```python
from build123d import *

# Parameters (mm, degrees)
SKETCH1_W           = 46
SKETCH1_H           = 6
BOSS_EXTRUDE1_DEPTH = 27.35
BOSS_EXTRUDE2_DEPTH = 27.35
FILLET1_R           = 7
BOSS_EXTRUDE3_DEPTH = 86
FILLET2_R           = 3
SKETCH5_R           = 8
SKETCH5_R_2         = 4
CUT_EXTRUDE1_DEPTH  = 116.185263628
SKETCH6_R           = 4
CUT_EXTRUDE2_DEPTH  = 116.185263741
SKETCH7_R           = 4
CUT_EXTRUDE3_DEPTH  = 116.185263741
SKETCH8_R           = 8
SKETCH8_R_2         = 4
BOSS_EXTRUDE4_DEPTH = 6
SKETCH9_R           = 8
SKETCH9_R_2         = 4
BOSS_EXTRUDE5_DEPTH = 6
SKETCH11_R          = 4
BOSS_EXTRUDE6_DEPTH = 3


with BuildPart() as part:
    # Sketch1 → Boss-Extrude1 (new body)
    with BuildSketch(Plane(origin=(0, 0, 0), x_dir=(0, 0, -1), z_dir=(1, 0, 0))):
        with Locations((1.147704591, 3)):
            Rectangle(SKETCH1_W, SKETCH1_H)
    extrude(amount=-BOSS_EXTRUDE1_DEPTH)

    # Sketch2 → Boss-Extrude2 (add)
    with BuildSketch(Plane(origin=(0, 0, 0), x_dir=(0, 0, -1), z_dir=(1, 0, 0))):
        Polygon((-21.852295409, 6), (-65.755273625, -10.778811155), (-63.703152765, -16.41696688), (-18.597906967, 0), align=None)
    extrude(amount=-BOSS_EXTRUDE2_DEPTH)

    # Fillet1
    fillet1_edges = [part.edges().sort_by_distance(p)[0] for p in [
        (-13.675, 6, 21.852295409),
    ]]
    fillet(fillet1_edges, radius=FILLET1_R)

    # Sketch3 → Boss-Extrude3 (add)
    with BuildSketch(Plane(origin=(0, 0, -24.147704591), x_dir=(-1, 0, 0), z_dir=(0, 0, -1))):
        with BuildLine():
            ThreePointArc((27.35, 6), (13.675, 19.675), (0, 6))
            Line((0, 6), (27.35, 6))
        make_face()
        with BuildLine():
            Line((25.963434603, 0), (1.386565397, 0))
            ThreePointArc((1.386565397, 0), (13.675, -7.675), (25.963434603, 0))
        make_face()
        with BuildLine():
            Line((27.35, 6), (0, 6))
            ThreePointArc((0, 6), (0.351149802, 2.920935061), (1.386565397, 0))
            Line((1.386565397, 0), (25.963434603, 0))
            ThreePointArc((25.963434603, 0), (26.998850198, 2.920935061), (27.35, 6))
        make_face()
    extrude(amount=BOSS_EXTRUDE3_DEPTH)

    # Fillet2
    # the kernel refuses this fillet: 3 mm, written as the material it adds along each edge
    with BuildSketch(Plane(origin=(0, 6, -24.147704591), x_dir=(0, 0, 1), z_dir=(-1, 0, 0))) as fillet2_piece_1_section:
        with BuildLine():
            CenterArc((FILLET2_R, FILLET2_R), FILLET2_R, 180, 90)
            Line((0, FILLET2_R), (0, 0))
            Line((0, 0), (FILLET2_R, 0))
        make_face()
    fillet2_piece_1 = extrude(amount=27.35, mode=Mode.PRIVATE)
    fillet2_piece_1 = fillet2_piece_1 & Plane(origin=(-13.675, 6, -23.467343504), x_dir=(-1, 0, 0), z_dir=(0, 0, 1)) * Cylinder(13.675, 67, mode=Mode.PRIVATE)
    add(fillet2_piece_1)

    # Sketch5 → Cut-Extrude1 (cut, through all)
    with BuildSketch(Plane(origin=(0, 0, 0), x_dir=(1, 0, 0), z_dir=(0, 1, 0))):
        with Locations(Location((-12.203148076, 67.147704591, 0), (0, 0, 259.398243128))):
            Circle(SKETCH5_R)
        with Locations(Location((-12.203148076, 67.147704591, 0), (0, 0, 248.409956221))):
            Circle(SKETCH5_R_2, mode=Mode.SUBTRACT)
    extrude(amount=CUT_EXTRUDE1_DEPTH, mode=Mode.SUBTRACT)

    # Sketch6 → Cut-Extrude2 (cut, through all)
    with BuildSketch(Plane(origin=(0, 0, 0), x_dir=(1, 0, 0), z_dir=(0, 1, 0))):
        with Locations((-12.203148076, 67.147704591)):
            Circle(SKETCH6_R)
    extrude(amount=CUT_EXTRUDE2_DEPTH, mode=Mode.SUBTRACT)

    # Sketch7 → Cut-Extrude3 (cut, through all)
    with BuildSketch(Plane(origin=(0, 0, 0), x_dir=(1, 0, 0), z_dir=(0, 1, 0))):
        with Locations(Location((-12.203148076, 67.147704591, 0), (0, 0, 270))):
            Circle(SKETCH7_R)
    extrude(amount=-CUT_EXTRUDE3_DEPTH, mode=Mode.SUBTRACT)

    # Sketch8 → Boss-Extrude4 (add)
    with BuildSketch(Plane(origin=(0, 0, 0), x_dir=(1, 0, 0), z_dir=(0, 1, 0))):
        with Locations(Location((-12.203148076, 67.147704591, 0), (0, 0, 259.398243128))):
            Circle(SKETCH8_R)
        with Locations(Location((-12.203148076, 67.147704591, 0), (0, 0, 270))):
            Circle(SKETCH8_R_2, mode=Mode.SUBTRACT)
    extrude(amount=BOSS_EXTRUDE4_DEPTH)

    # Sketch9 → Boss-Extrude5 (add)
    with BuildSketch(Plane(origin=(0, 6, 0), x_dir=(1, 0, 0), z_dir=(0, 1, 0))):
        with Locations(Location((-12.203148076, 67.147704591, 0), (0, 0, 259.398243128))):
            Circle(SKETCH9_R)
        with Locations(Location((-12.203148076, 67.147704591, 0), (0, 0, 270))):
            Circle(SKETCH9_R_2, mode=Mode.SUBTRACT)
    extrude(amount=BOSS_EXTRUDE5_DEPTH)


with BuildPart() as part_1:
    # Body-Move/Copy1: moved
    add(part.part.moved(Location((13.675, 0, 0))))

    # Sketch11 → Boss-Extrude6 (add, symmetric)
    with BuildSketch(Plane(origin=(0, 0, 0), x_dir=(0, 0, -1), z_dir=(1, 0, 0))):
        with BuildLine():
            Line((-65.755273625, -10.778811155), (-21.830832444, 5.883719563))
            Line((-21.830832444, 5.883719563), (-26.796391829, 18.97353316))
            ThreePointArc((-26.796391829, 18.97353316), (-28.894991358, 21.202538099), (-31.955069824, 21.294748649))
            Line((-31.955069824, 21.294748649), (-68.432005738, 7.457394118))
            ThreePointArc((-68.432005738, 7.457394118), (-70.663039196, 5.354278937), (-70.749698163, 2.289463448))
            Line((-70.749698163, 2.289463448), (-65.755273625, -10.778811155))
        make_face()
        with Locations((-43.013345846, 5.334970097)):
            Circle(SKETCH11_R, mode=Mode.SUBTRACT)
    extrude(amount=BOSS_EXTRUDE6_DEPTH, both=True)


solid = part_1.part
```
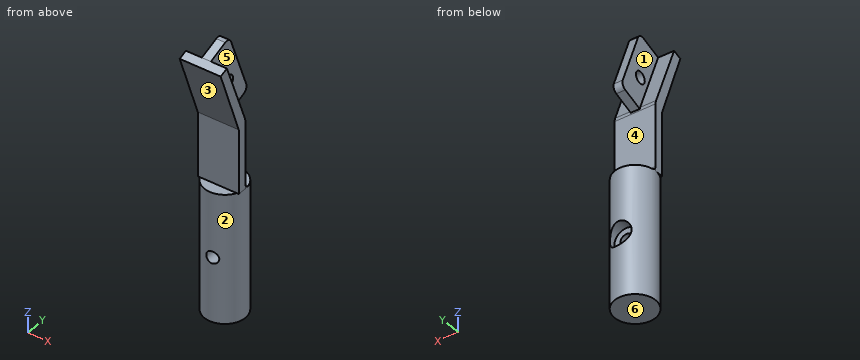
Input: part model. Units: mm. Frame: model coordinates. Face numbers are marked on the shaded views. A direction names the side the tool comes from. Give positions to 0.01 mm unless a question says otherwise; leave off trailing zeros. Write each loop counter-clockwise with the first axis right and the second up, starting at its lowest first coordinate (ties: lowest second). Pieces come first, ordered by that corner, then holes. Notation, with made-up numbers: (-13, 37) - (40, 37) arc R22 ccw to (40, 47) - close; hole circle Ø4 at (-37.75, 60.5). An arc over 180 degrees is marked (long way). Write item = value, one per line. Start each with the question number.
1) Reachability of the marked faces 1, 2 and 3 from +Z, -Z, +X, -X, +Y, -Y: full face, straight path, thin tool, end or side. Return the list, or none.
2) Cut plane D-D (x = -8.25). Return loops of the section in (y, z), and give its area (3 significant figures).
3) Cut plane B-B (y = 17). Return loops of the section in (x, z), and give its area (3 significant figures).
4) Cut plane C-C (z = -52). Return loops of the section in (x, y) (3 decimals), and give its area (3 significant figures).
5) Pin query (flat end, axial travel): pin 1 (2 mm diameter, centred on x = 7, y = -6.5, fed in from -Z); pin 2 (5 mm diameter, centred on x = 4, z = -21, fed in from -Y); pin 3 (10.5 mm diameter, centred on x = 1.47, z = -67.15, fed in from +Y); pin 4 (5 mm diameter, centred on x = 3.5, z = 34.5, fed in from -Y). Return the tip coordinate at first contact, or that it passes through.
6) Draft query along Z for the marked faces 4, 5 and 6. Return one class per face: pulls with the +Z half, pulls with the -Z half, needs draft (parallel to the pull), parting line crosses it, or undercut.
7) Material intervals for L1, parallel to X at y = 3, z = 34; L2, parallel to Z at x = -12, y = 11; L3, parallel to Y at x = 1, z = 18.5, sorted ascending. Write a range as [from, to].
8) Cut plane A-A (y = -4.5). Return loops of the section in (x, z) (3 decimals), and give its area (3 significant figures).
Answers follow:
q1.face_1 = +Z, -X, +Y
q1.face_2 = -Z
q1.face_3 = +X, -X, -Y
q2.outline = (-16.42, 63.7) - (0, 18.6) - (0, -24.15) - (-4.91, -24.15) - (-4.91, -110.15) - (16.91, -110.15) - (16.91, -24.15) - (9, -24.15) arc R3 cw to (6, -21.15) - (6, 20.56) arc R7 ccw to (5.54, 23.06) - (-10.78, 65.76) - close
q2.area = 2,450 mm^2
q3.outline = (-8.12, -110.15) - (8.12, -110.15) - (8.12, -71.59) arc R8 cw (long way) to (8.12, -62.7) - (8.12, -24.15) - (-8.12, -24.15) - close; (-3, 26.05) - (3, 26.05) - (3, 43.28) - (-3, 43.28) - close
q3.area = 1,310 mm^2
q4.outline = circle Ø27.35 at (0, 6)
q4.area = 587 mm^2
q5.pin_1 = -110.15
q5.pin_2 = 0
q5.pin_3 = 12
q5.pin_4 = -6.7
q6.face_4 = undercut
q6.face_5 = needs draft
q6.face_6 = pulls with the -Z half
q7.L1 = [-3, 3]
q7.L2 = [-110.15, -24.15]
q7.L3 = [0, 6]
q8.outline = (-13.675, 30.962) - (13.675, 30.962) - (13.675, 49.326) - (3, 49.326) - (3, 68.155) - (-3, 68.155) - (-3, 49.326) - (-13.675, 49.326) - close; (-8.761, -110.148) - (8.761, -110.148) - (8.761, -24.148) - (-8.761, -24.148) - close; hole circle Ø8 at (1.472, -67.148)
q8.area = 2,070 mm^2
